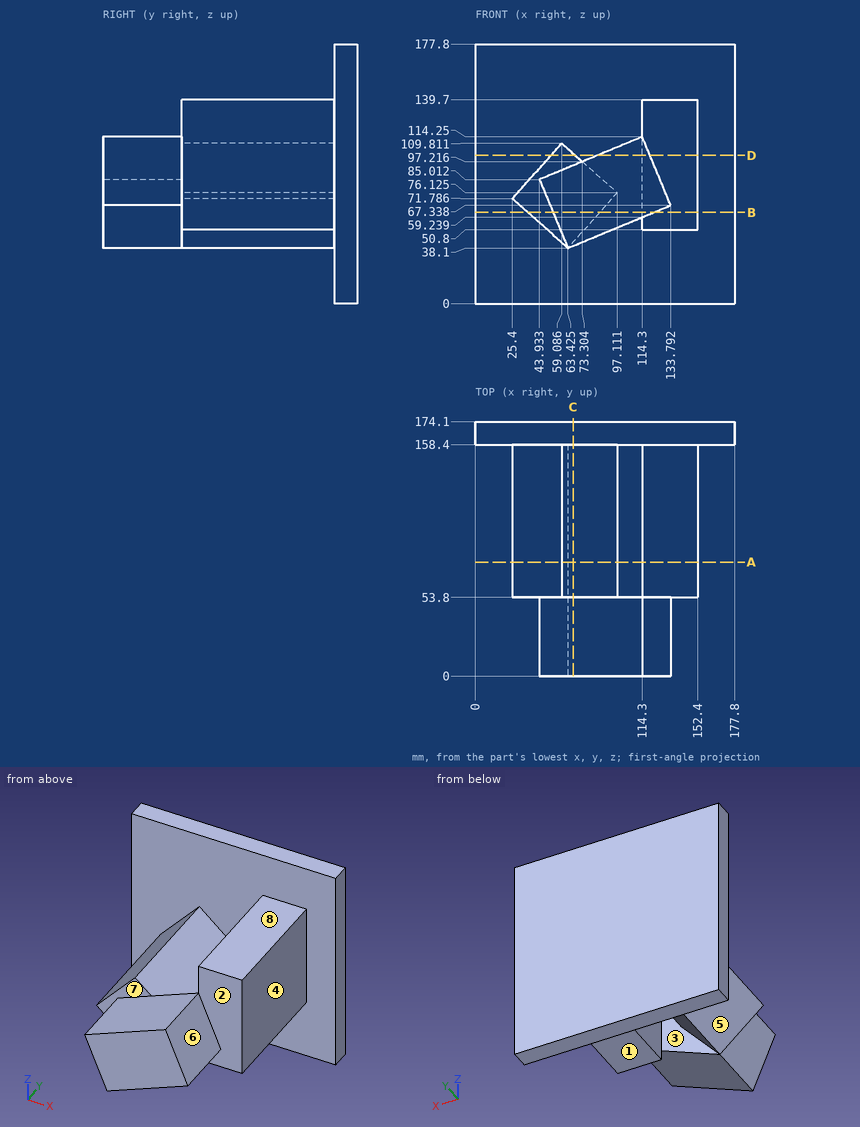
The figure shows three views and two pictorial views of one solid part (mm, origin at its lowest corner). Answer the questions. A direction names the side the tool comes from. Give positions to 0.01 mm unless a question says otherwise; leave off trailing zeros. Loops run counter-clockwise (first coordinate to the right, second up) from the corner with the lowest first, then second, coordinate; pieces in that order, holes last. Notation, with made-up numbers: M 45,2.25 L 54,2.25 A28 cw 54,28.25 Z; hole C -21.75,-39 d6. An arc over 180 degrees is marked long. Write each question's results on one line, items separated by ' | '.
1. Given pin 1 (10 mm diameter, centred on x = 109.5, y = 144.5, fed in from -Z); pin 2 (2 mm diameter, centred on y = 87, z = 71, fed in from -X); pin 3 (2 mm diameter, centred on y = 126, z = 110.5, fed in from -X), each flat-ended and moving along its own axis, determine where each tip first touches the part or whether it passes through.
Values:
pin 1: stops at z = 50.8 | pin 2: stops at x = 25.4 | pin 3: stops at x = 58.81
2. A tool of negligible diameter and unlimited length cuts with its end or side. For the marked faces 4, 5, 6, 7 and 8, from which of +Z, -Z, +X, -X, +Y, -Y can it reach the whole face along a straight path? Write none if from no direction.
Values:
face 4: +Z, -Z, +X, -Y | face 5: -Z, -X, -Y | face 6: +Z, +X, -Y | face 7: -X, -Y | face 8: +Z, +X, -X, -Y
3. Section B-B on z = 62.5 is taken. Give the vertices of the cut face in (x, y), plus the area to 3 significant figures.
Values:
outline: M 0,158.4 L 35.88,158.4 L 35.88,53.8 L 53.29,53.8 L 53.29,0 L 122.15,0 L 122.15,53.8 L 152.4,53.8 L 152.4,158.4 L 177.8,158.4 L 177.8,174.1 L 0,174.1 Z; hole M 85.04,53.8 L 114.3,53.8 L 114.3,158.4 L 85.04,158.4 Z | area: 15,600 mm^2
4. Section C-C on x = 67 is taken. Give the vertices of the cut face in (y, z) (1 decimal).
Values:
outline: M 0,39.6 L 53.8,39.6 L 53.8,42.1 L 158.4,42.1 L 158.4,0 L 174.1,0 L 174.1,177.8 L 158.4,177.8 L 158.4,102.8 L 53.8,102.8 L 53.8,94.6 L 0,94.6 Z
5. Section D-D on z = 101.5 is taken. Give the vertices of the cut face in (x, y) (1 decimal), plus the area to 3 significant figures.
Values:
outline: M 0,158.4 L 51.7,158.4 L 51.7,53.8 L 68.5,53.8 L 68.5,158.4 L 114.3,158.4 L 114.3,53.8 L 83.6,53.8 L 83.6,0 L 119.6,0 L 119.6,53.8 L 152.4,53.8 L 152.4,158.4 L 177.8,158.4 L 177.8,174.1 L 0,174.1 Z | area: 10,500 mm^2
6. The mould has two halves that part along Y. Classify the marked faces 1, 2 and 3: pulls with the +Y half, pulls with the -Y half, needs draft (parallel to the pull), parting line crosses it, or undercut.
Values:
face 1: needs draft | face 2: pulls with the -Y half | face 3: undercut
7. Section A-A on y = 78 is taken. Give the vertices of the cut face in (x, z) (1 decimal).
Values:
outline: M 25.4,71.8 L 63.4,38.1 L 97.1,76.1 L 59.1,109.8 Z; M 114.3,50.8 L 152.4,50.8 L 152.4,139.7 L 114.3,139.7 Z
8. Straight lines are drawn through the part: line 1 (Y direction, x = 77, z = 45); line 2 (Y direction, x = 47.5, z = 96.5); line 3 (Y direction, x = 49, z = 135). For each, find the intervals that lie inside material, in ascending order. Write a range as [from, to].
Values:
line 1: y = [0, 53.8], [158.4, 174.1] | line 2: y = [53.8, 174.1] | line 3: y = [158.4, 174.1]
